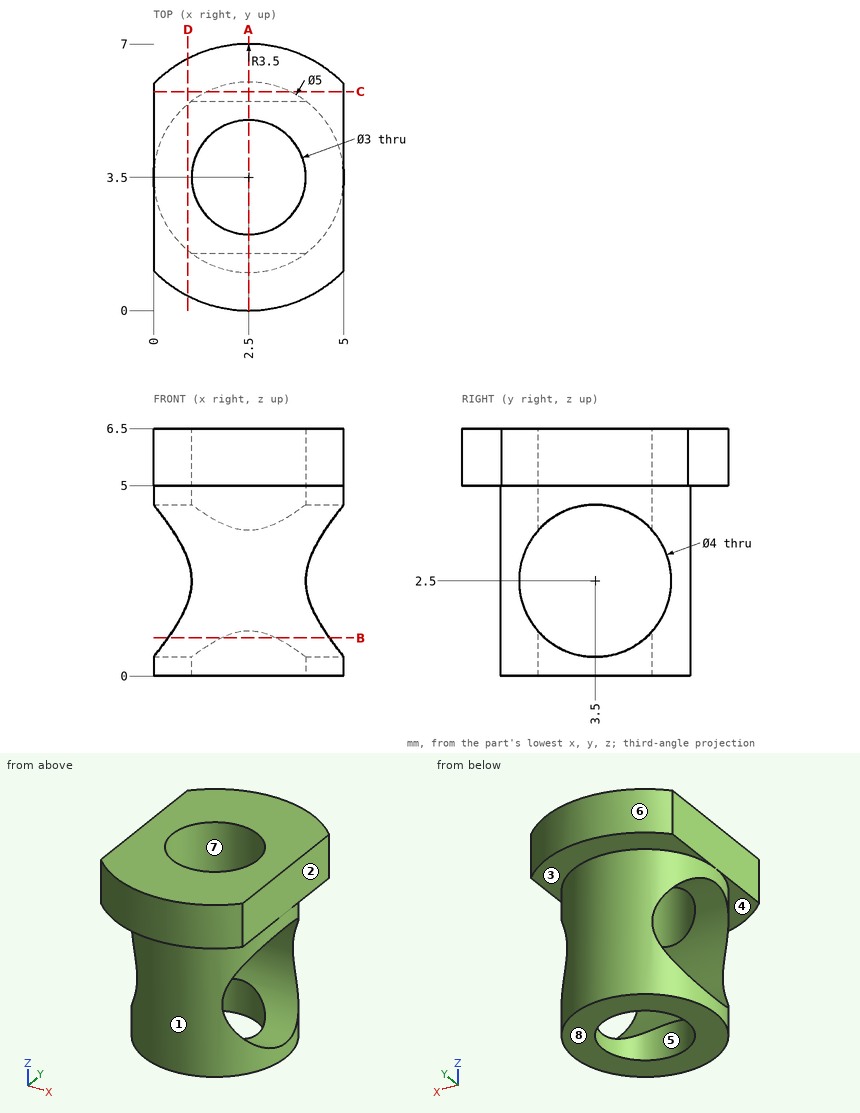
Drawing for the job (mm, zero at the part's lowest x, y, z). A direction names the side the tool comes from. Round coordinates to 2 decimals unless told otherwise and drop trailing zeros. Write each loop counter-clockwise with the first axis right and the second up, starting at its lowest first coordinate (ties: lowest second). Pieces come first, ordered by that corner, then holes. Notation, with made-up numbers: M 45.5,84 L 71.5,84 A18 cw 71.5,102 Z; hole C 67.5,-6 d4. An arc over 180 degrees is marked long. Answer as a JSON object with one key per item and string values. Group by question number.
(1) Cut at C-C (y = 5.75). Give the cut face in (x, z), and give its area (3 significant figures).
(2) Flat gauge pins, fed straight in: pin 1 (1 mm diameter, centred on y = 5, z = 4, fed in from -X); pin 2 (1 mm diameter, centred on x = 1.5, z = 2.5, fed in from -Y); pin 3 (1 mm diameter, centred on x = 4.5, z = 3, fed in from +Y). Where does each tip first touch, or does it go through?
(3) Cut at D-D (x = 0.9). Give the cut face in (y, z), and give its area (3 significant figures).
(4) Drill centre lines: L1, parallel to Z at x = 3.35, y = 2; L2, parallel to Z at x = 2.25, y = 6.25; L3, parallel to Y at x = 2.55, z = 2.5. Where is each one in solid material? Low to high.
(5) Cut at A-A (x = 2.5). Give the cut face in (y, z).
(6) Which spindle directions (+Z, -Z, +X, -X, +Y, -Y) get a long thin tool onto all of the face, cutting with end or side? Do the marked faces 1, 2, 3 and 4. Say none if no direction does.
(7) Mould opens along X. For the marked faces 5, 6, 7 and 8 say: pulls with the +X half, pulls with the -X half, needs draft (parallel to the pull), parting line crosses it, or undercut.
(8) Cut at B-B (z = 1). Give the cut face in (x, y), and give its area (3 significant figures).
Responses:
{
 "1": {"outline": "M 0,5 L 1.41,5 L 1.41,0 L 3.59,0 L 3.59,5 L 5,5 L 5,6.5 L 0,6.5 Z", "area": "18.4 mm2"},
 "2": {"pin 1": "stops at x = 0.23", "pin 2": "stops at y = 1.05", "pin 3": "stops at y = 5.5"},
 "3": {"outline": "M 0.39,5 L 1.58,5 L 1.58,3.06 A2 cw 5.42,3.06 L 5.42,5 L 6.61,5 L 6.61,6.5 L 0.39,6.5 Z; M 1.58,0 L 5.42,0 L 5.42,1.94 A2 cw 1.58,1.94 Z", "area": "16.1 mm2"},
 "4": {"L1": "z = 0 to 1.18, 3.82 to 6.5", "L2": "z = 5 to 6.5", "L3": "y = 1 to 1.5, 5.5 to 6"},
 "5": {"outline": "M 0,5 L 1,5 L 1,0 L 2,0 L 2,1.18 A2 cw 2,3.82 L 2,6.5 L 0,6.5 Z; M 5,0 L 6,0 L 6,5 L 7,5 L 7,6.5 L 5,6.5 L 5,3.82 A2 cw 5,1.18 Z"},
 "6": {"face 1": "-Z", "face 2": "+Z, -Z, +X, +Y, -Y", "face 3": "-Z, +Y", "face 4": "-Z, -Y"},
 "7": {"face 5": "undercut", "face 6": "parting line crosses it", "face 7": "undercut", "face 8": "needs draft"},
 "8": {"outline": "M 0.38,2.18 A2.5 ccw 4.62,2.18 L 3.21,2.18 A1.5 cw 1.79,2.18 Z; M 0.38,4.82 L 1.79,4.82 A1.5 cw 3.21,4.82 L 4.62,4.82 A2.5 ccw Z", "area": "6.71 mm2"}
}
